```python
from build123d import *

# Parameters (mm, degrees)
F0_W     = 273.6599
F0_H     = 130.27117
F0_W_2   = 38.90042
F0_H_2   = 42.066727
F0_W_3   = 47.042365
F0_H_3   = 28.949149
F0_W_4   = 31.663131
F0_H_4   = 37.091095
F0_W_5   = 27.592152
F0_H_5   = 26.687497
F0_W_6   = 42.519059
F0_H_6   = 42.519063
F1_DEPTH = 25.4


with BuildPart() as f1:
    # F0 (on Front) → F1 (new body)
    with BuildSketch(Plane.XZ):
        with Locations((-2.035491, -16.283898)):
            Rectangle(F0_W, F0_H)
        with Locations((-87.752104, -51.339505)):
            Rectangle(F0_W_2, F0_H_2, mode=Mode.SUBTRACT)
        with Locations((13.569912, -49.756351)):
            Rectangle(F0_W_3, F0_H_3, mode=Mode.SUBTRACT)
        with Locations((-34.377114, 4.070974)):
            Rectangle(F0_W_4, F0_H_4, mode=Mode.SUBTRACT)
        with Locations((-110.142462, 19.224043)):
            Rectangle(F0_W_5, F0_H_5, mode=Mode.SUBTRACT)
        with Locations((73.277535, -2.261653)):
            Rectangle(F0_W_6, F0_H_6, mode=Mode.SUBTRACT)
    extrude(amount=F1_DEPTH)


solid = f1.part
```
Geometry: final body of the model. Coordinates: model frame, mm. A direction names the side the tool comes from. Round coordinates to 2 decimals unless told otherwise and drop trailing zeros. Order: outer loops, then holes, each group sorted by start corner. A loop starts at its lowest first (then second) coordinate and runs counter-clockwise, first axis right, second up. Notation, with made-up numbers: (-22, -40) -> (-3, -40) arc R21 cw to (-3, -10) -> close; hole circle Ø1 at (-34.75, 15). An arc over 180 degrees is marked (long way). Use CSV: the item, a comma, the result in double quotes. Start each with the question number.
1) Section D-D (z = -6). Return the cut outline in (x, y).
2) Section C-C (y = -5.25). Return the cut outline in (x, z).
3) Set-up query: faces 1 (the face through (134.794, -13, -17)), 2 (the face through (-110, -13, 5.88)). Return all of +Z, -Z, +X, -X, +Y, -Y with unobstructed straight access to the full face (end or side cutting, diameter ignored); none if empty.
4) Section A-A (x = -29). Return the cut outline in (y, z), and give its area (3 significant figures).
5) Section B-B (z = -69.5). Return the cut outline in (x, y).
6) Material intervals for line 1 along X through (y, z) = (-7.75, -3.5); line 2 along X through (y, z) = (-9, 16.5); line 3 along Z through (x, y) = (-107, -13.25), sorted ascending. Write a range as from..to.
7) Draft query along Z for faces 3 (the face through (-4, 0, -15)), 4 (the face through (-4, -13, -81.419)), 5 (the face through (-35, -13, 22.617)). Return one class per face: +Z half, -Z half, draft (parallel to the pull), parting line (faces both ways), or undercut.
Returned:
1,outline,"(-138.87, -25.4) -> (-50.21, -25.4) -> (-50.21, 0) -> (-138.87, 0) -> close; (-18.55, -25.4) -> (52.02, -25.4) -> (52.02, 0) -> (-18.55, 0) -> close; (94.54, -25.4) -> (134.79, -25.4) -> (134.79, 0) -> (94.54, 0) -> close"
2,outline,"(-138.87, -81.42) -> (134.79, -81.42) -> (134.79, 48.85) -> (-138.87, 48.85) -> close; hole (-123.94, 5.88) -> (-96.35, 5.88) -> (-96.35, 32.57) -> (-123.94, 32.57) -> close; hole (-107.2, -72.37) -> (-68.3, -72.37) -> (-68.3, -30.31) -> (-107.2, -30.31) -> close; hole (-50.21, -14.47) -> (-18.55, -14.47) -> (-18.55, 22.62) -> (-50.21, 22.62) -> close; hole (-9.95, -64.23) -> (37.09, -64.23) -> (37.09, -35.28) -> (-9.95, -35.28) -> close; hole (52.02, -23.52) -> (94.54, -23.52) -> (94.54, 19) -> (52.02, 19) -> close"
3,face 1,"+Z, -Z, +X, +Y, -Y"
3,face 2,"+Y, -Y"
4,outline,"(-25.4, -81.42) -> (0, -81.42) -> (0, -14.47) -> (-25.4, -14.47) -> close; (-25.4, 22.62) -> (0, 22.62) -> (0, 48.85) -> (-25.4, 48.85) -> close"
4,area,"2,370 mm²"
5,outline,"(-138.87, -25.4) -> (-107.2, -25.4) -> (-107.2, 0) -> (-138.87, 0) -> close; (-68.3, -25.4) -> (134.79, -25.4) -> (134.79, 0) -> (-68.3, 0) -> close"
6,line 1,"x = -138.87..-50.21, -18.55..52.02, 94.54..134.79"
6,line 2,"x = -138.87..-123.94, -96.35..-50.21, -18.55..52.02, 94.54..134.79"
6,line 3,"z = -81.42..-72.37, -30.31..5.88, 32.57..48.85"
7,face 3,"draft"
7,face 4,"-Z half"
7,face 5,"undercut"
